```python
from build123d import *

# Parameters (mm, degrees)
SKETCH1_W           = 32.142857143
SKETCH1_H           = 6.35
SKETCH1_W_2         = 32.142857142
BOSS_EXTRUDE1_DEPTH = 6.35
SKETCH2_W           = 212.3
SKETCH2_H           = 112.5
CUT_EXTRUDE1_DEPTH  = 314.804310041
SKETCH3_W           = 212.3
SKETCH3_H           = 17.5
CUT_EXTRUDE2_DEPTH  = 6.35
SKETCH4_W           = 6.35
SKETCH4_H           = 18.05999894
SKETCH4_H_2         = 20.32
SKETCH4_H_3         = 14.71000106
BOSS_EXTRUDE2_DEPTH = 6.35
SKETCH5_W           = 183
SKETCH5_H           = 73.156
CUT_EXTRUDE3_DEPTH  = 245.316029969
SKETCH6_W           = 225
SKETCH6_H           = 6.35
BOSS_EXTRUDE3_DEPTH = 6.35
SKETCH7_W           = 5.08
SKETCH7_H           = 6.35
SKETCH7_W_2         = 26.14
CUT_EXTRUDE4_DEPTH  = 245.316029969


with BuildPart() as part:
    # Sketch1 → Boss-Extrude1 (new body)
    with BuildSketch(Plane(origin=(0, 0, 0), x_dir=(1, 0, 0), z_dir=(0, 1, 0))):
        Polygon((6.35, 6.35), (32.142857143, 6.35), (64.285714286, 6.35), (96.428571429, 6.35), (128.571428571, 6.35), (160.714285714, 6.35), (192.857142857, 6.35), (218.65, 6.35), (218.65, 32.142857143), (218.65, 64.285714286), (218.65, 96.428571429), (218.65, 128.571428571), (218.65, 160.714285714), (218.65, 192.857142857), (218.65, 218.65), (192.857142857, 218.65), (160.714285714, 218.65), (128.571428571, 218.65), (96.428571429, 218.65), (64.285714286, 218.65), (32.142857143, 218.65), (6.35, 218.65), (6.35, 192.857142857), (6.35, 160.714285714), (6.35, 128.571428571), (6.35, 96.428571429), (6.35, 64.285714286), (6.35, 32.142857143), align=None)
        with Locations((48.214285715, 221.825)):
            Rectangle(SKETCH1_W, SKETCH1_H)
        with Locations((112.5, 221.825)):
            Rectangle(SKETCH1_W_2, SKETCH1_H)
        with Locations((176.785714286, 221.825)):
            Rectangle(SKETCH1_W, SKETCH1_H)
        with Locations((176.785714286, 3.175)):
            Rectangle(SKETCH1_W, SKETCH1_H)
        with Locations((112.5, 3.175)):
            Rectangle(SKETCH1_W_2, SKETCH1_H)
        with Locations((48.214285715, 3.175)):
            Rectangle(SKETCH1_W, SKETCH1_H)
    extrude(amount=BOSS_EXTRUDE1_DEPTH)

    # Sketch2 → Cut-Extrude1 (cut, through all)
    with BuildSketch(Plane(origin=(0, 6.35, 0), x_dir=(1, 0, 0), z_dir=(0, 1, 0))):
        with Locations((112.5, 168.75)):
            Rectangle(SKETCH2_W, SKETCH2_H)
    extrude(amount=-CUT_EXTRUDE1_DEPTH, mode=Mode.SUBTRACT)

    # Sketch3 → Cut-Extrude2 (cut)
    with BuildSketch(Plane(origin=(0, 6.35, 0), x_dir=(1, 0, 0), z_dir=(0, 1, 0))):
        with Locations((112.5, 103.75)):
            Rectangle(SKETCH3_W, SKETCH3_H)
    extrude(amount=-CUT_EXTRUDE2_DEPTH, mode=Mode.SUBTRACT)

    # Sketch4 → Boss-Extrude2 (add)
    with BuildSketch(Plane(origin=(0, 6.35, 0), x_dir=(1, 0, 0), z_dir=(0, 1, 0))):
        with Locations((3.175, 85.97000053)):
            Rectangle(SKETCH4_W, SKETCH4_H)
        with Locations((3.175, 61.70000106)):
            Rectangle(SKETCH4_W, SKETCH4_H_2)
        with Locations((3.175, 36.30000106)):
            Rectangle(SKETCH4_W, SKETCH4_H_2)
        with Locations((3.175, 13.70500053)):
            Rectangle(SKETCH4_W, SKETCH4_H_3)
        with Locations((221.825, 85.97000053)):
            Rectangle(SKETCH4_W, SKETCH4_H)
        with Locations((221.825, 61.70000106)):
            Rectangle(SKETCH4_W, SKETCH4_H_2)
        with Locations((221.825, 36.30000106)):
            Rectangle(SKETCH4_W, SKETCH4_H_2)
        with Locations((221.825, 13.70500053)):
            Rectangle(SKETCH4_W, SKETCH4_H_3)
    extrude(amount=-BOSS_EXTRUDE2_DEPTH)

    # Sketch5 → Cut-Extrude3 (cut, through all)
    with BuildSketch(Plane.XZ):
        with Locations((112.5, -58.422)):
            Rectangle(SKETCH5_W, SKETCH5_H)
    extrude(amount=-CUT_EXTRUDE3_DEPTH, mode=Mode.SUBTRACT)

    # Sketch6 → Boss-Extrude3 (add)
    with BuildSketch(Plane.XZ):
        with Locations((112.5, -3.175)):
            Rectangle(SKETCH6_W, SKETCH6_H)
    extrude(amount=-BOSS_EXTRUDE3_DEPTH)

    # Sketch7 → Cut-Extrude4 (cut, through all)
    with BuildSketch(Plane.XZ):
        with Locations((176, -3.175)):
            Rectangle(SKETCH7_W, SKETCH7_H)
        with Locations((150.6, -3.175)):
            Rectangle(SKETCH7_W, SKETCH7_H)
        with Locations((125.2, -3.175)):
            Rectangle(SKETCH7_W, SKETCH7_H)
        with Locations((99.8, -3.175)):
            Rectangle(SKETCH7_W, SKETCH7_H)
        with Locations((74.4, -3.175)):
            Rectangle(SKETCH7_W, SKETCH7_H)
        with Locations((49, -3.175)):
            Rectangle(SKETCH7_W, SKETCH7_H)
        with Locations((211.93, -3.175)):
            Rectangle(SKETCH7_W_2, SKETCH7_H)
        with Locations((13.07, -3.175)):
            Rectangle(SKETCH7_W_2, SKETCH7_H)
    extrude(amount=-CUT_EXTRUDE4_DEPTH, mode=Mode.SUBTRACT)


solid = part.part
```
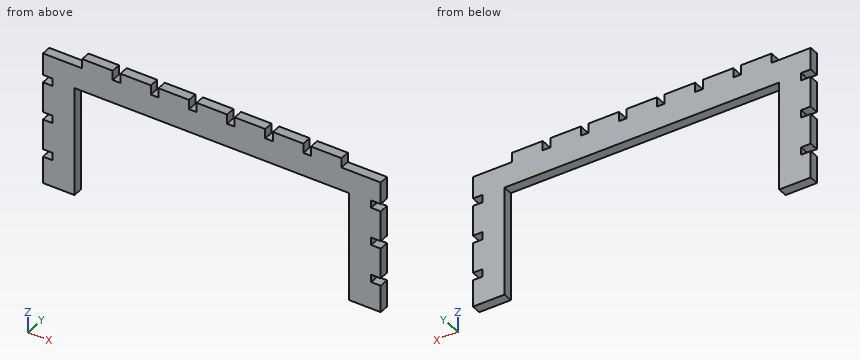
The listing builds one solid part. Answer for the finished solid, in the listing's coordinates (mm). Coordinates: 2 decimals unless noted, no trailing zeros. Write each loop counter-clockwise with the first axis right and the second up, starting at its lowest first coordinate (ties: lowest second). Pieces come first, ordered by that corner, then holes.
Q1. Section C-C, the plane x = 185 is taken. Write down the section's boundary in (y, z).
Returned:
outline: (0, -21.84) - (6.35, -21.84) - (6.35, 0) - (0, 0) - close
Q2. Given P1, Ø3, axis at y = 2, z = -2, coming from the +X side; P2, Ø3, axis at y = 4, z = -2.5, coming from the -X side; P3, Ø1.5, axis at y = 2.5, z = -74, coming from the -X side, each flat-ended and moving along its own axis, determine where each tip first touches the part or whether it passes through.
Returned:
P1: stops at x = 198.86
P2: stops at x = 26.14
P3: stops at x = 6.35
Q3. Section B-B, the plane x = 125 is taken. Write down the section's boundary in (y, z).
Returned:
outline: (0, -21.84) - (6.35, -21.84) - (6.35, -6.35) - (0, -6.35) - close
Q4. Section A-A, the plane z = -30 is taken. Write down the section's boundary in (x, y), then the cut area to 3 significant figures.
Returned:
outline: (0, 0) - (21, 0) - (21, 6.35) - (0, 6.35) - close; (204, 0) - (225, 0) - (225, 6.35) - (204, 6.35) - close
area: 267 mm2
Q5. Find the intervals of material crossed by line 1 along X through (y, z) = (1.75, -87.5); line 2 along X through (y, z) = (4, -51.5); line 3 along Z through (x, y) = (176.5, 2.25), in increasing order.
Returned:
line 1: x = 0 to 21, 204 to 225
line 2: x = 6.35 to 21, 204 to 218.65
line 3: z = -21.84 to -6.35
